Input: dimensioned drawing with shaded views. Units: mm. Origin: part minimum x, y, z. A direction names the side the tool comes from. Round coordinates to 2 decimals unless told otherwise and drop trailing zeros. Order: outer loops, then holes, each group sorted by start corner. A loop starts at its lowest first (then second) coordinate and runs counter-clockwise, first axis right, second up.
Item 1: Reachability of the marked faces 1 and 2 from +Z, -Z, +X, -X, +Y, -Y: full face, straight path, thin tool, end or side. Return the list, or none.
Item 2: Cut plane C-C on y = 6. Output: boundary loops of the cut face in (x, z).
Item 3: Cut plane B-B on z = 27.5. Output: boundary loops of the cut face in (x, y), then the cut area to 3 significant figures.
Item 4: Mould query, pull axis Z, two halves, no side actions, for the marked faces 3, 4, 5 and 6. Classes: released by +Z, released by -Z, zero draft, split by the parting line, or undercut.
Item 5: Cut plane D-D on x = 33. Output: boundary loops of the cut face in (y, z).
Item 6: First-contact query: pin 1 (2 mm diameter, centred on x = 46.5, z = 8, fed in from +Y); pin 2 (4 mm diameter, centred on y = 6, z = 28, fed in from +X). Flat tips, straight axial feed; report the tip coordinate or a pass-through.
Item 7: Line query: L1, parallel to X at y = 8.35, z = 46; L2, parallel to Z at x = 9, y = 7.45; L3, parallel to Z at x = 46, y = 8.45. Output: solid intervals per line, ascending.
Item 8: Cut plane A-A on x = 46. Output: boundary loops of the cut face in (y, z).
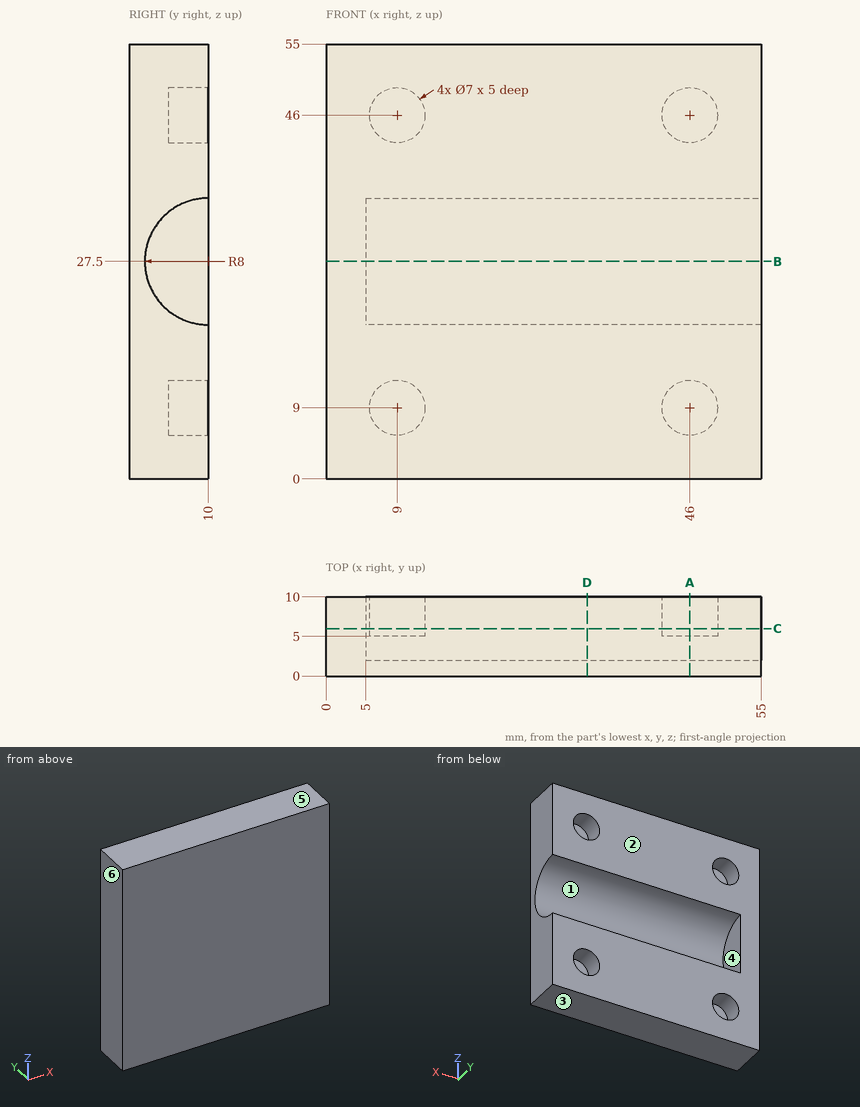
From the geometry:
1. face 1: +X, +Y
1. face 2: +Z, -Z, +X, -X, +Y
2. outline: (0, 0) - (55, 0) - (55, 20.57) - (5, 20.57) - (5, 34.43) - (55, 34.43) - (55, 55) - (0, 55) - close; hole circle Ø7 at (9, 9); hole circle Ø7 at (9, 46); hole circle Ø7 at (46, 9); hole circle Ø7 at (46, 46)
3. outline: (0, 0) - (55, 0) - (55, 2) - (5, 2) - (5, 10) - (0, 10) - close
3. area: 150 mm2
4. face 3: released by -Z
4. face 4: undercut
4. face 5: released by +Z
4. face 6: zero draft
5. outline: (0, 0) - (10, 0) - (10, 19.5) arc R8 cw to (10, 35.5) - (10, 55) - (0, 55) - close
6. pin 1: stops at y = 5
6. pin 2: stops at x = 5
7. L1: x = 0 to 5.5, 12.5 to 42.5, 49.5 to 55
7. L2: z = 0 to 5.5, 12.5 to 19.92, 35.08 to 42.5, 49.5 to 55
7. L3: z = 0 to 5.5, 12.5 to 19.65, 35.35 to 42.5, 49.5 to 55
8. outline: (0, 0) - (10, 0) - (10, 5.5) - (5, 5.5) - (5, 12.5) - (10, 12.5) - (10, 19.5) arc R8 cw to (10, 35.5) - (10, 42.5) - (5, 42.5) - (5, 49.5) - (10, 49.5) - (10, 55) - (0, 55) - close
